The model under review builds one solid part; all positions refer to its coordinate system, in mm. A direction names the side the tool comes from. Round coordinates to 2 decimals unless told otherwise and drop trailing zeros. Write each loop counter-clockwise with the first axis right and the second up, starting at its lowest first coordinate (ties: lowest second). Pieces come first, ordered by that corner, then holes. Notation, with made-up numbers: M -13.5,82 L 23.5,82 A13 ccw 23.5,88 Z; hole C 61.25,-16 d10. An arc over 180 degrees is marked long. Write item = value, one per line. Start each with the question number.
Item 1: Take a section at C-C, the plane y = 7. Give the boundary of the cut face in (x, z), plus the area to 3 significant figures.
Item 2: To check wall thickness, follow line 1 along X through (y, z) = (4, -23); line 2 along Z through (x, y) = (25, 9.5); line 3 along Y through (x, z) = (28, -51.5). State the ranges of each line that lie inside material, in increasing order.
Item 3: Take a section at A-A, the plane x = 16. Give the boundary of the cut face in (y, z), plus the area to 3 significant figures.
Item 4: Take a section at B-B, the plane y = 13.5. Give the boundary of the cut face in (x, z), plus the area to 3 significant figures.
Item 5: Tool access review of faces 1 (the flat face through (2.5, 14, -42)), 2 (the flat face through (3, 12, -40)), 3 (the flat face through (10, 1, -46.111)), 4 (the flat face through (2.5, 14, -11)): name each direction out of +Z, -Z, +X, -X, +Y, -Y from which nothing blocks a thin tool from reaching the whole face with its end or side.
Item 6: The part is to be moulded in two halves that separate along Y. For faces 5 (the flat face through (29, 7, -28)), 6 (the flat face through (15, 0, -35)), 7 (the flat face through (28.5, 15, -47)), 8 (the flat face through (2, 14, -40)), say which applies: +Y half, -Y half, draft (parallel to the pull), parting line (faces both ways), or undercut.
Item 7: For pin 1 Ø2 at (y, z) = (12, -46) entering from -X; pin 2 Ø1 at (x, z) = (25.5, -24.5) entering from +Y; pin 3 Ø0.5 at (x, y) = (2.5, 13.5) entering from +Z, all flat-tipped, find the tip position at first contact; note any pin that passes through.
Item 8: Take a section at D-D, the plane z = -13. Give the boundary of the cut face in (x, y), plus the area to 3 significant figures.
from build123d import *

# Parameters (mm, degrees)
ESQUISSE1_W             = 31
ESQUISSE1_H             = 56
BOSS_EXTRU_1_DEPTH      = 2
ENL_V_MAT_EXTRU_1_DEPTH = 65.039050586
ESQUISSE6_W             = 31
ESQUISSE6_H             = 56
ESQUISSE6_W_2           = 27
ESQUISSE6_H_2           = 52
BOSS_EXTRU_3_DEPTH      = 10
ESQUISSE10_W            = 4
ESQUISSE10_H            = 6
BOSS_EXTRU_8_DEPTH      = 1
CONG_1_R                = 1
ESQUISSE11_W            = 4
ESQUISSE11_H            = 6
BOSS_EXTRU_11_DEPTH     = 1
CONG_2_R                = 1


with BuildPart() as part:
    # Esquisse1 → Boss.-Extru.1 (new body)
    with BuildSketch(Plane(origin=(0, 0, 0), x_dir=(1, 0, 0), z_dir=(0, 1, 0))):
        with Locations((15.5, 28)):
            Rectangle(ESQUISSE1_W, ESQUISSE1_H)
    extrude(amount=BOSS_EXTRU_1_DEPTH)

    # Esquisse2 → Enlèv. mat.-Extru.1 (cut, through all)
    with BuildSketch(Plane(origin=(0, 2, 0), x_dir=(1, 0, 0), z_dir=(0, 1, 0))):
        Polygon((13.380581824, 43.489934015), (11.867381431, 46.110873977), (8.840980645, 46.110873977), (7.327780252, 43.489934015), (8.840980645, 40.868994052), (11.867381431, 40.868994052), align=None)
        Polygon((13.380581824, 26.792968516), (11.867381431, 29.413908479), (8.840980645, 29.413908479), (7.327780252, 26.792968516), (8.840980645, 24.172028553), (11.867381431, 24.172028553), align=None)
        Polygon((18.526400786, 46.460873977), (17.013200393, 49.08181394), (13.986799607, 49.08181394), (12.473599214, 46.460873977), (13.986799607, 43.839934015), (17.013200393, 43.839934015), align=None)
        Polygon((18.526400786, 40.518994052), (17.013200393, 43.139934015), (13.986799607, 43.139934015), (12.473599214, 40.518994052), (13.986799607, 37.898054089), (17.013200393, 37.898054089), align=None)
        Polygon((23.672219675, 43.490211012), (22.158779402, 46.111012465), (19.132378628, 46.110735468), (17.619418128, 43.489657017), (19.132858402, 40.868855564), (22.159259175, 40.869132561), align=None)
        Polygon((18.526400786, 29.763908479), (17.013200393, 32.384848442), (13.986799607, 32.384848442), (12.473599214, 29.763908479), (13.986799607, 27.142968516), (17.013200393, 27.142968516), align=None)
        Polygon((18.526400786, 23.822028553), (17.013200393, 26.442968516), (13.986799607, 26.442968516), (12.473599214, 23.822028553), (13.986799607, 21.20108859), (17.013200393, 21.20108859), align=None)
        Polygon((23.672219675, 26.793245513), (22.158779402, 29.414046967), (19.132378628, 29.413769969), (17.619418128, 26.792691519), (19.132858402, 24.171890065), (22.159259175, 24.172167063), align=None)
    extrude(amount=-ENL_V_MAT_EXTRU_1_DEPTH, mode=Mode.SUBTRACT)

    # Esquisse6 → Boss.-Extru.3 (add)
    with BuildSketch(Plane(origin=(0, 2, 0), x_dir=(1, 0, 0), z_dir=(0, 1, 0))):
        with Locations((15.5, 28)):
            Rectangle(ESQUISSE6_W, ESQUISSE6_H)
        with Locations((15.5, 28)):
            Rectangle(ESQUISSE6_W_2, ESQUISSE6_H_2, mode=Mode.SUBTRACT)
    extrude(amount=BOSS_EXTRU_3_DEPTH)

    # Esquisse10 → Boss.-Extru.8 (add)
    with BuildSketch(Plane.ZY.offset(-29)):
        with Locations((-47, 12)):
            Rectangle(ESQUISSE10_W, ESQUISSE10_H)
        with Locations((-9, 12)):
            Rectangle(ESQUISSE10_W, ESQUISSE10_H)
    extrude(amount=BOSS_EXTRU_8_DEPTH)

    # Congé1
    cong_1_edges = [part.edges().sort_by_distance(p)[0] for p in [
        (29, 9, -9),
        (29, 10.5, -11),
        (29, 10.5, -7),
        (29, 9, -47),
        (29, 10.5, -45),
        (29, 10.5, -49),
    ]]
    fillet(cong_1_edges, radius=CONG_1_R - 0.0001)  # a hair under: the kernel refuses the full size

    # Esquisse11 → Boss.-Extru.11 (add)
    with BuildSketch(Plane(origin=(2, 0, 0), x_dir=(0, 0, -1), z_dir=(1, 0, 0))):
        with Locations((9, 12)):
            Rectangle(ESQUISSE11_W, ESQUISSE11_H)
        with Locations((40, 12)):
            Rectangle(ESQUISSE11_W, ESQUISSE11_H)
    extrude(amount=BOSS_EXTRU_11_DEPTH)

    # Congé2
    cong_2_edges = [part.edges().sort_by_distance(p)[0] for p in [
        (2, 10.5, -7),
        (2, 9, -9),
        (2, 10.5, -11),
        (2, 10.5, -42),
        (2, 9, -40),
        (2, 10.5, -38),
    ]]
    fillet(cong_2_edges, radius=CONG_2_R - 0.0001)  # a hair under: the kernel refuses the full size


solid = part.part
Response values:
q1.outline = M 0,-56 L 31,-56 L 31,0 L 0,0 Z; hole M 2,-54 L 29,-54 L 29,-2 L 2,-2 Z
q1.area = 332 mm2
q2.line_1 = 0 to 2, 29 to 31
q2.line_2 = -56 to -54, -2 to 0
q2.line_3 = 0 to 2
q3.outline = M 0,-56 L 12,-56 L 12,-54 L 2,-54 L 2,-49.08 L 0,-49.08 Z; M 0,-43.84 L 2,-43.84 L 2,-43.14 L 0,-43.14 Z; M 0,-37.9 L 2,-37.9 L 2,-32.38 L 0,-32.38 Z; M 0,-27.14 L 2,-27.14 L 2,-26.44 L 0,-26.44 Z; M 0,-21.2 L 2,-21.2 L 2,-2 L 12,-2 L 12,0 L 0,0 Z
q3.area = 110 mm2
q4.outline = M 2,-42 L 3,-42 L 3,-38 L 2,-38 Z; M 2,-11 L 3,-11 L 3,-7 L 2,-7 Z; M 28,-49 L 29,-49 L 29,-45 L 28,-45 Z; M 28,-11 L 29,-11 L 29,-7 L 28,-7 Z
q4.area = 16.0 mm2
q5.face_1 = -Z, +X, -X, +Y
q5.face_2 = +Y
q5.face_3 = +Y, -Y
q5.face_4 = +X, -X, +Y
q6.face_5 = undercut
q6.face_6 = -Y half
q6.face_7 = +Y half
q6.face_8 = draft
q7.pin_1 = 0
q7.pin_2 = 2
q7.pin_3 = -7
q8.outline = M 0,0 L 31,0 L 31,12 L 29,12 L 29,2 L 2,2 L 2,12 L 0,12 Z
q8.area = 102 mm2
